Here's how the part is built. I have some questions about the finished solid (model axes, mm). Face numbers are marked on the shaded views. A direction names the side the tool comes from. Round coordinates to 2 decimals unless told otherwise and drop trailing zeros. Use a Markdown table: item, result.
from build123d import *

# Parameters (mm, degrees)
SKETCH2_R          = 51
CUT_EXTRUDE1_DEPTH = 400
SKETCH3_R          = 33
SKETCH3_R_2        = 3.1
CUT_EXTRUDE2_DEPTH = 40
SKETCH3_2_R        = 3.1
CUT_EXTRUDE4_DEPTH = 617.757438246


with BuildPart() as part:
    # Sketch1 → Revolve1 (revolve)
    with BuildSketch(Plane.XY, mode=Mode.PRIVATE) as revolve1_sk:
        with BuildLine():
            Line((650, 78.36), (600, 78.36))
            add(Edge.make_bspline(
                [(200, 42.32828037), (208.17052038, 43.513954023), (225.684887064, 45.995278148), (252.564625249, 49.617202919), (288.837779512, 54.154525537), (326.320734141, 58.489281574), (363.841177133, 62.486312126), (401.395994208, 66.14650922), (438.982971251, 69.460608736), (476.600652971, 72.407109383), (509.54226569, 74.628697811), (537.796481139, 76.233504653), (560.29226218, 77.275459401), (575.195356704, 77.83264328), (587.214225045, 78.173006727), (594.519976189, 78.310355882), (598.17325676, 78.35432466), (600, 78.36)],
                knots=[0.337827743, 0.337827743, 0.337827743, 0.337827743, 0.337827743, 0.392246706, 0.454423417, 0.516600127, 0.57877684, 0.640953552, 0.703130263, 0.765306975, 0.827483687, 0.889660399, 0.920748755, 0.951837111, 0.975918556, 0.987959278, 1, 1, 1, 1, 1], degree=4))
            Line((200, 42.32828037), (200, 0))
            Line((200, 0), (806.72, 0))
            Line((806.72, 0), (806.72, 55))
            Line((806.72, 55), (650, 55))
            Line((650, 55), (650, 78.36))
        make_face()
    revolve(revolve1_sk.sketch.rotate(Axis((806.72, 0, 0), (-1, 0, 0)), 90), axis=Axis((806.72, 0, 0), (-1, 0, 0)))

    # Sketch2 → Cut-Extrude1 (cut)
    with BuildSketch(Plane(origin=(806.72, 0, 0), x_dir=(0, 0, -1), z_dir=(1, 0, 0))):
        Circle(SKETCH2_R)
    extrude(amount=-CUT_EXTRUDE1_DEPTH, mode=Mode.SUBTRACT)

    # Sketch3 → Cut-Extrude2 (cut)
    with BuildSketch(Plane.ZY.offset(-200)):
        Circle(SKETCH3_R)
        with Locations((0, 20)):
            Circle(SKETCH3_R_2, mode=Mode.SUBTRACT)
        with Locations((0, -20)):
            Circle(SKETCH3_R_2, mode=Mode.SUBTRACT)
    extrude(amount=-CUT_EXTRUDE2_DEPTH, mode=Mode.SUBTRACT)

    # Sketch3_2 → Cut-Extrude4 (cut, through all)
    with BuildSketch(Plane.ZY.offset(-200)):
        with Locations((0, 20)):
            Circle(SKETCH3_2_R)
        with Locations((0, -20)):
            Circle(SKETCH3_2_R)
    extrude(amount=-CUT_EXTRUDE4_DEPTH, mode=Mode.SUBTRACT)


solid = part.part
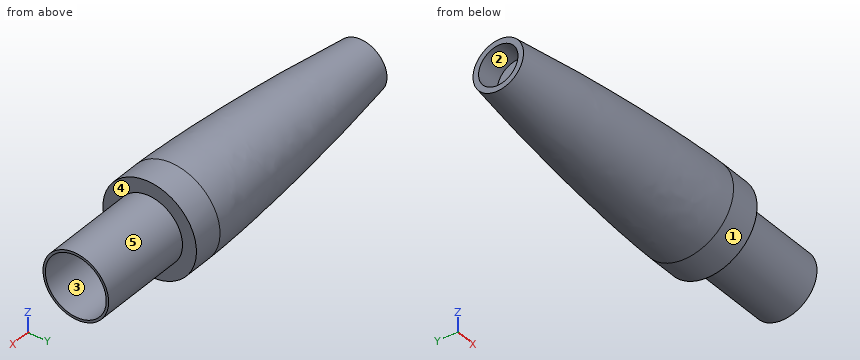
1. Imagine slicing it at A-A, the plane x = 271. State how many separate pieces and enclosed holes the cut face has, then the cut area to 3 significant figures.
Answer sheet:
| item | result |
|---|---|
| separate pieces | 1 |
| enclosed holes | 2 |
| area | 8,400 mm2 |
2. We'd pull the mould along Z, two halves only. Please class the marked faces 3, 4 and 5: +Z half, -Z half, draft (parallel to the pull), parting line (faces both ways), or undercut.
Answer sheet:
| item | result |
|---|---|
| face 3 | undercut |
| face 4 | draft |
| face 5 | parting line |
3. Which directions (+Z, -Z, +X, -X, +Y, -Y) give clear straight access to the entire face, cutting with the end or side of a thin tool? Please do the marked faces 1 and 2.
Answer sheet:
| item | result |
|---|---|
| face 1 | +X, -X |
| face 2 | -X |
4. For pin 1 Ø10 at (y, z) = (-20, 0) entering from -X; pin 2 Ø10 at (x, z) = (304.5, -30.5) entering from +Y; pin 3 Ø10 at (x, z) = (573, 33.5) entering from -Y; pin 4 Ø5 at (y, z) = (20, 0) entering from -X, each with a flat end and sliding along its axis, tell me the tip position at first contact or that it passes through.
Answer sheet:
| item | result |
|---|---|
| pin 1 | x = 240 |
| pin 2 | y = 49.87 |
| pin 3 | y = -72.33 |
| pin 4 | through |
5. I need wall thicknesses on probe 1 along Y at (x, z) = (318, 0); probe 2 along X at (y, z) = (17.5, 35); probe 3 along Y at (x, z) = (518, -22). Which ranges of each line are inside material? Lowest first, please. Write a range as from..to.
Answer sheet:
| item | result |
|---|---|
| probe 1 | -57.49..-23.1, -16.9..16.9, 23.1..57.49 |
| probe 2 | 200..406.72 |
| probe 3 | -71.78..-46.01, 46.01..71.78 |
